For this review, use the dimensioned drawing (mm, ordinates from the lowest corner) and the shaded views. A direction names the side the tool comes from. Coordinates: 2 decimals unless noted, no trailing zeros. Write each loop counter-clockwise with the first axis right and the second up, starting at its lowest first coordinate (ties: lowest second). Pieces come first, ordered by that corner, then holes. Notation, with made-up numbers: (-26.75, 78.5) -> (-8.75, 78.5) arc R22 cw to (-8.75, 84.5) -> close; hole circle Ø2 at (19.5, -28.5). An arc over 180 degrees is marked (long way). Return JSON: item names as keys, results as strings. Group by question number.
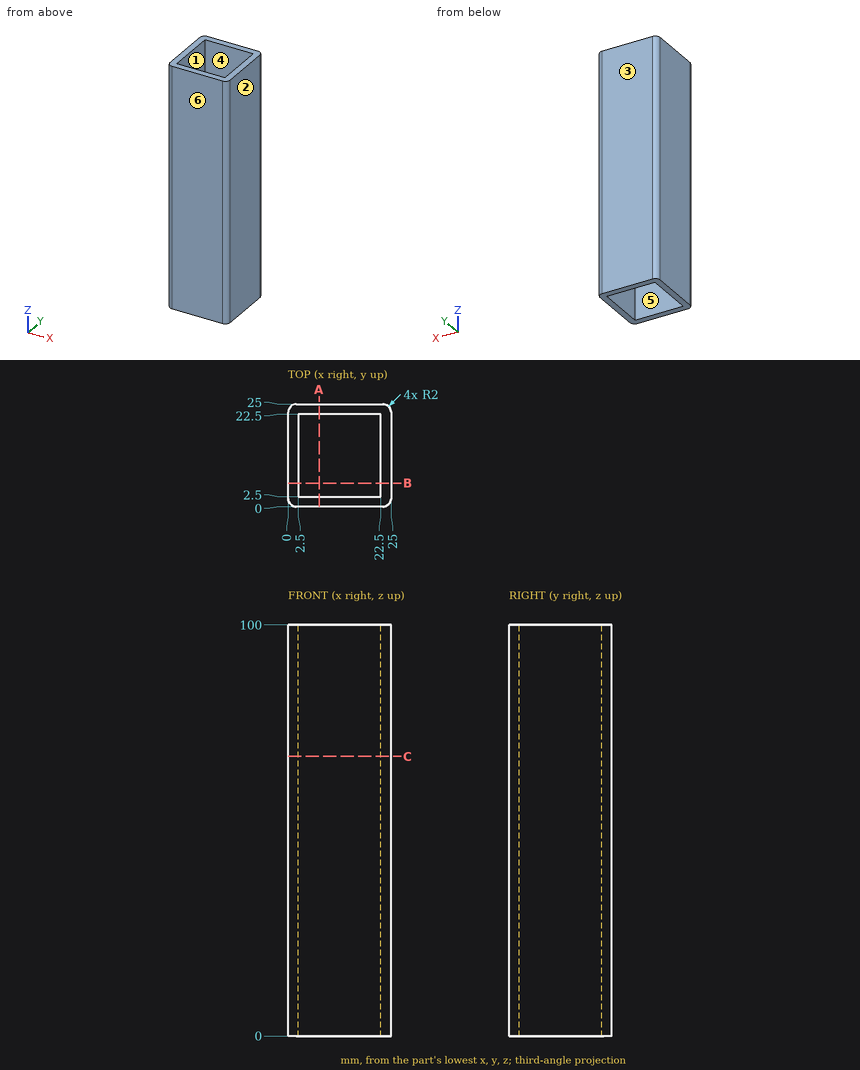
Q1. Wall thickness on L1, parallel to Y at x = 12.75, z = 14.5; L2, parallel to Y at x = 23.5, z = 90: over which ranges is each line inside the solid? List them lowest first.
Q2. For the marked faces 5 and 6, list the 3-axis set-ups (+Z, -Z, +X, -X, +Y, -Y) from which the entire face can be reached by the end or side of a thin tool; tool diameter is ignored.
Q3. We need section C-C on z = 68. Write out the cut boundary in (x, y).
Q4. The part is to be moulded in two halves that separate along X. For the marked faces 1, 2, 3 and 4, say which applies: +X half, -X half, draft (parallel to the pull), parting line (faces both ways), or undercut.
Q5. We need section A-A on x = 7.5. Write out the cut boundary in (y, z).
Findings below:
{
 "1": {"L1": "y = 0 to 2.5, 22.5 to 25", "L2": "y = 0.06 to 24.94"},
 "2": {"face 5": "+Z, -Z", "face 6": "+Z, -Z, +X, -X, -Y"},
 "3": {"outline": "(0, 2) arc R2 ccw to (2, 0) -> (23, 0) arc R2 ccw to (25, 2) -> (25, 23) arc R2 ccw to (23, 25) -> (2, 25) arc R2 ccw to (0, 23) -> close; hole (2.5, 2.5) -> (22.5, 2.5) -> (22.5, 22.5) -> (2.5, 22.5) -> close"},
 "4": {"face 1": "undercut", "face 2": "+X half", "face 3": "draft", "face 4": "undercut"},
 "5": {"outline": "(0, 0) -> (2.5, 0) -> (2.5, 100) -> (0, 100) -> close; (22.5, 0) -> (25, 0) -> (25, 100) -> (22.5, 100) -> close"}
}
